For this review, take the finished solid that the model builds, in its own axes (mm). A direction names the side the tool comes from. Round coordinates to 2 decimals unless told otherwise and drop trailing zeros. Order: outer loops, then holes, each group sorted by start corner. A loop starts at its lowest first (then second) coordinate and runs counter-clockwise, first axis right, second up. Notation, with made-up numbers: (14, -28) -> (67, -28) arc R6 ccw to (67, -18) -> close; hole circle Ø10 at (26.5, 8.25). An arc over 180 degrees is marked (long way). Use a Markdown table: item, result. Add a question column.
1) Machinability: for faces 4 (the face through (-72.979, -24.995, 13.97)), 5 (the face through (7.014, -173, 14)), 6 (the face through (4.514, -173, 14)), which of the approach directions +Z, -Z, +X, -X, +Y, -Y give a long, thin tool a straight path to every point of the face, cutting with its end or side? Answer none if there is none.
2) Consider section B-B (y = -228.5). State the section outline as (x, z) points, plus the area to 4 significant figures.
3) Consider section C-C (x = -14.5). State the section outline as (y, z) points.
4) Draft analysis for pull direction X (two halves, no side actions). For faces 1 (the face through (-35, -173, 27.5)), 2 (the face through (-35, -173, 2.5)), 3 (the face through (6.12, -344.13, 13.56)), state which applies: pulls with the +X half, pulls with the -X half, needs draft (parallel to the pull), parting line crosses it, or undercut.
5) Consider section A-A (z = 21.75). State the section outline as (x, y) points.
6) Clearance check with flat-ended pins moving along their axes: P1, Ø4, axis at x = -58, z = 3, coming from the +Y side; P2, Ø6, axis at y = -20, z = 13.75, coming from the +X side. State where each tip first meets the part, or that it passes through.
7) Wall thickness on line 1 along Z through (x, y) = (-72.75, -20); line 2 along Z through (x, y) = (-72, -20); line 3 along X through (y, z) = (-273, 7.5): over which ranges is each line inside the solid? List them lowest first. Write a range as [from, to].
8) Consider section D-D (y = -20). State the section outline as (x, z) points, plus the area to 4 significant figures.
```python
from build123d import *

# Parameters (mm, degrees)
F0_W        = 82
F0_H        = 27.5
F0_W_2      = 77
F0_H_2      = 22.5
F1_DEPTH    = 350
F3_DEPTH    = 53
F4_T1_DEPTH = 77.5
F5_R        = 5
F6_DEPTH    = 80.5


# Not quite as in the source:
# - a fillet or chamfer that OpenCascade refuses, or shapes differently, is made with other operations: its cross-section is extruded or revolved along the edge and cut away or added
# - a feature names something its author has since deleted; it is built from what else it names


with BuildPart() as f1:
    # F0 (on Front) → F1 (new body)
    with BuildSketch(Plane.XZ):
        with Locations((-33.9858543277, 13.75)):
            Rectangle(F0_W, F0_H)
        with Locations((-33.9858543277, 13.75)):
            Rectangle(F0_W_2, F0_H_2, mode=Mode.SUBTRACT)
    extrude(amount=F1_DEPTH)

    # F2 (on Top) → F3 (cut)
    with BuildSketch(Plane.XY):
        with BuildLine():
            Line((-59.9858543277, -340), (-59.9858543277, -335))
            ThreePointArc((-59.9858543277, -335), (-64.9858543277, -340), (-59.9858543277, -345))
            Line((-59.9858543277, -345), (-59.9858543277, -340))
        make_face()
        with BuildLine():
            ThreePointArc((-54.9858543277, -340), (-56.4503204217, -336.4644660941), (-59.9858543277, -335))
            Line((-59.9858543277, -335), (-59.9858543277, -340))
            Line((-59.9858543277, -340), (-59.9858543277, -345))
            ThreePointArc((-59.9858543277, -345), (-56.4503204217, -343.5355339059), (-54.9858543277, -340))
        make_face()
        with BuildLine():
            Line((-59.9858543277, -45), (-59.9858543277, -35))
            ThreePointArc((-59.9858543277, -35), (-64.9858543277, -40), (-59.9858543277, -45))
        make_face()
        with BuildLine():
            ThreePointArc((-54.9858543277, -40), (-56.4503204217, -36.4644660941), (-59.9858543277, -35))
            Line((-59.9858543277, -35), (-59.9858543277, -45))
            ThreePointArc((-59.9858543277, -45), (-56.4503204217, -43.5355339059), (-54.9858543277, -40))
        make_face()
        with BuildLine():
            Line((-59.9858543277, -15), (-59.9858543277, -5))
            ThreePointArc((-59.9858543277, -5), (-64.9858543277, -10), (-59.9858543277, -15))
        make_face()
        with BuildLine():
            ThreePointArc((-59.9858543277, -15), (-56.4503204217, -13.5355339059), (-54.9858543277, -10))
            ThreePointArc((-54.9858543277, -10), (-56.4503204217, -6.4644660941), (-59.9858543277, -5))
            Line((-59.9858543277, -5), (-59.9858543277, -15))
        make_face()
        with BuildLine():
            Line((-59.9858543277, -315), (-59.9858543277, -305))
            ThreePointArc((-59.9858543277, -305), (-64.9858543277, -310), (-59.9858543277, -315))
        make_face()
        with BuildLine():
            ThreePointArc((-54.9858543277, -310), (-56.4503204217, -306.4644660941), (-59.9858543277, -305))
            Line((-59.9858543277, -305), (-59.9858543277, -315))
            ThreePointArc((-59.9858543277, -315), (-56.4503204217, -313.5355339059), (-54.9858543277, -310))
        make_face()
    extrude(amount=F3_DEPTH, mode=Mode.SUBTRACT)

    # F4: fillet of radius 10 on 4 edges, made by hand

    # F4_s2 → F4_t1 (cut)
    with BuildSketch(Plane.XY.offset(-25)):
        with BuildLine():
            ThreePointArc((-64.9858543277, 0), (-72.0569221395, -2.9289321881), (-74.9858543277, -10))
            Line((-74.9858543277, -10), (-74.9858543277, 0))
            Line((-74.9858543277, 0), (-64.9858543277, 0))
        make_face()
        with BuildLine():
            ThreePointArc((-64.9858543277, -350), (-72.0569221395, -347.0710678119), (-74.9858543277, -340))
            Line((-74.9858543277, -340), (-74.9858543277, -350))
            Line((-74.9858543277, -350), (-64.9858543277, -350))
        make_face()
        with BuildLine():
            ThreePointArc((7.0141456723, -10), (4.0852134842, -2.9289321881), (-2.9858543277, 0))
            Line((-2.9858543277, 0), (7.0141456723, 0))
            Line((7.0141456723, 0), (7.0141456723, -10))
        make_face()
        with BuildLine():
            ThreePointArc((7.0141456723, -340), (4.0852134842, -347.0710678119), (-2.9858543277, -350))
            Line((-2.9858543277, -350), (7.0141456723, -350))
            Line((7.0141456723, -350), (7.0141456723, -340))
        make_face()
    extrude(amount=F4_T1_DEPTH, mode=Mode.SUBTRACT)

    # F5 (on face) → F6 (cut)
    with BuildSketch(Plane.YZ.offset(7.0141456723)):
        with Locations((-20, 13.75)):
            Circle(F5_R)
    extrude(amount=-F6_DEPTH, mode=Mode.SUBTRACT)


solid = f1.part
```
Results list:
| question | item | result |
|---|---|---|
| 1 | face 4 | +X |
| 1 | face 5 | +Z, -Z, +X, +Y, -Y |
| 1 | face 6 | +Y, -Y |
| 2 | outline | (-74.99, 0) -> (7.01, 0) -> (7.01, 27.5) -> (-74.99, 27.5) -> close; hole (-72.49, 2.5) -> (4.51, 2.5) -> (4.51, 25) -> (-72.49, 25) -> close |
| 2 | area | 522.5 mm2 |
| 3 | outline | (-350, 0) -> (0, 0) -> (0, 2.5) -> (-350, 2.5) -> close; (-350, 25) -> (0, 25) -> (0, 27.5) -> (-350, 27.5) -> close |
| 4 | face 1 | needs draft |
| 4 | face 2 | undercut |
| 4 | face 3 | pulls with the +X half |
| 5 | outline | (-74.99, -340) arc R10 ccw to (-72.49, -346.61) -> (-72.49, -3.39) arc R10 ccw to (-74.99, -10) -> close; (4.51, -346.61) arc R10 ccw to (7.01, -340) -> (7.01, -10) arc R10 ccw to (4.51, -3.39) -> close |
| 6 | P1 | y = 0 |
| 6 | P2 | x = -73.49 |
| 7 | line 1 | [0, 8.75], [18.75, 27.5] |
| 7 | line 2 | [0, 2.5], [25, 27.5] |
| 7 | line 3 | [-74.99, -72.49], [4.51, 7.01] |
| 8 | outline | (-74.99, 0) -> (7.01, 0) -> (7.01, 8.75) -> (4.51, 8.75) -> (4.51, 2.5) -> (-72.49, 2.5) -> (-72.49, 8.75) -> (-73.49, 8.75) -> (-73.49, 18.75) -> (-72.49, 18.75) -> (-72.49, 25) -> (4.51, 25) -> (4.51, 18.75) -> (7.01, 18.75) -> (7.01, 27.5) -> (-74.99, 27.5) -> close |
| 8 | area | 487.5 mm2 |
